from build123d import *

# Parameters (mm, degrees)
F0_R     = 3.175
F1_DEPTH = 3.048


with BuildPart() as f1:
    # F0 (on Front) → F1 (new body)
    with BuildSketch(Plane.XZ):
        with BuildLine():
            ThreePointArc((3.175, 0), (-2.2450640303, -2.2450640303), (0, 3.175))
            Line((0, 3.175), (0, 7.9375))
            ThreePointArc((0, 7.9375), (-6.000186009, 5.1963135112), (-7.8560875915, -1.1339285714))
            ThreePointArc((-7.8560875915, -1.1339285714), (-5.1963135112, -6.000186009), (0, -7.9375))
            ThreePointArc((0, -7.9375), (5.6126600757, -5.6126600757), (7.9375, 0))
            Line((7.9375, 0), (3.175, 0))
        make_face()
        with BuildLine():
            ThreePointArc((-7.8560875915, -1.1339285714), (-6.000186009, 5.1963135112), (0, 7.9375))
            Line((0, 7.9375), (0, 39.6875))
            ThreePointArc((0, 39.6875), (-10.3926270225, 43.562127982), (-15.7121751829, 53.2946428571))
            Line((-15.7121751829, 53.2946428571), (-7.8560875915, -1.1339285714))
        make_face()
        with BuildLine():
            Line((0, 39.6875), (0, 7.9375))
            ThreePointArc((0, 7.9375), (5.6126600757, 5.6126600757), (7.9375, 0))
            Line((7.9375, 0), (36.5125, 0))
            ThreePointArc((36.5125, 0), (38.8373399243, 5.6126600757), (44.45, 7.9375))
            Line((44.45, 7.9375), (18.3455357436, 7.9375))
            ThreePointArc((18.3455357436, 7.9375), (12.335749437, 10.6830723871), (10.476878412, 17.0234428571))
            Line((10.476878412, 17.0234428571), (15.7121751829, 53.2946428571))
            ThreePointArc((15.7121751829, 53.2946428571), (10.3926270225, 43.562127982), (0, 39.6875))
        make_face()
        with BuildLine():
            Line((36.5125, 0), (7.9375, 0))
            ThreePointArc((7.9375, 0), (5.6126600757, -5.6126600757), (0, -7.9375))
            Line((0, -7.9375), (44.45, -7.9375))
            ThreePointArc((44.45, -7.9375), (38.8373399243, -5.6126600757), (36.5125, 0))
        make_face()
        with BuildLine():
            ThreePointArc((-15.7121751829, 53.2946428571), (-10.3926270225, 43.562127982), (0, 39.6875))
            Line((0, 39.6875), (0, 52.3875))
            ThreePointArc((0, 52.3875), (-3.175, 55.5625), (0, 58.7375))
            Line((0, 58.7375), (0, 71.4375))
            ThreePointArc((0, 71.4375), (-10.6011956271, 67.3790255586), (-15.7819589391, 57.2787159089))
            ThreePointArc((-15.7819589391, 57.2787159089), (-15.8725653423, 55.284481195), (-15.7121751829, 53.2946428571))
        make_face()
        with BuildLine():
            Line((0, 52.3875), (0, 39.6875))
            ThreePointArc((0, 39.6875), (10.3926270225, 43.562127982), (15.7121751829, 53.2946428571))
            ThreePointArc((15.7121751829, 53.2946428571), (15.8342414727, 54.4256526112), (15.875, 55.5625))
            ThreePointArc((15.875, 55.5625), (15.8517226608, 56.4218681903), (15.7819589056, 57.2787162162))
            ThreePointArc((15.7819589056, 57.2787162162), (10.601195512, 67.3790256618), (0, 71.4375))
            Line((0, 71.4375), (0, 58.7375))
            ThreePointArc((0, 58.7375), (2.2450640303, 57.8075640303), (3.175, 55.5625))
            ThreePointArc((3.175, 55.5625), (2.2450640303, 53.3174359697), (0, 52.3875))
        make_face()
        with BuildLine():
            ThreePointArc((44.45, 7.9375), (38.8373399243, 5.6126600757), (36.5125, 0))
            ThreePointArc((36.5125, 0), (38.8373399243, -5.6126600757), (44.45, -7.9375))
            ThreePointArc((44.45, -7.9375), (50.0626600757, -5.6126600757), (52.3875, 0))
            ThreePointArc((52.3875, 0), (50.0626600757, 5.6126600757), (44.45, 7.9375))
        make_face()
        with BuildLine():
            ThreePointArc((47.625, 0), (44.45, -3.175), (41.275, 0))
            ThreePointArc((41.275, 0), (44.45, 3.175), (47.625, 0))
        make_face(mode=Mode.SUBTRACT)
        with BuildLine():
            Line((-9.4691753434, 115.3297297297), (-15.7819589391, 57.2787159089))
            ThreePointArc((-15.7819589391, 57.2787159089), (-10.6011956271, 67.3790255586), (0, 71.4375))
            Line((0, 71.4375), (0, 88.7612230935))
            Line((0, 88.7612230935), (0, 104.775))
            ThreePointArc((0, 104.775), (-7.0899153971, 107.9392826928), (-9.4691753434, 115.3297297297))
        make_face()
        with Locations((-3.175, 88.7612230935)):
            Circle(F0_R, mode=Mode.SUBTRACT)
        with BuildLine():
            Line((0, 88.7612230935), (0, 71.4375))
            ThreePointArc((0, 71.4375), (10.601195512, 67.3790256618), (15.7819589056, 57.2787162162))
            Line((15.7819589056, 57.2787162162), (9.4691753434, 115.3297297297))
            ThreePointArc((9.4691753434, 115.3297297297), (9.5110335965, 114.8156209142), (9.525, 114.3))
            ThreePointArc((9.525, 114.3), (6.7351920908, 107.5648079092), (0, 104.775))
            Line((0, 104.775), (0, 88.7612230935))
        make_face()
        with BuildLine():
            ThreePointArc((9.4691753434, 115.3297297297), (0, 123.825), (-9.4691753434, 115.3297297297))
            ThreePointArc((-9.4691753434, 115.3297297297), (-7.0899153971, 107.9392826928), (0, 104.775))
            ThreePointArc((0, 104.775), (6.7351920908, 107.5648079092), (9.525, 114.3))
            ThreePointArc((9.525, 114.3), (9.5110335965, 114.8156209142), (9.4691753434, 115.3297297297))
        make_face()
        with BuildLine():
            ThreePointArc((3.175, 114.3), (2.2450640303, 112.0549359697), (0, 111.125))
            ThreePointArc((0, 111.125), (-2.2450640303, 116.5450640303), (3.175, 114.3))
        make_face(mode=Mode.SUBTRACT)
    extrude(amount=F1_DEPTH)


solid = f1.part
The listing builds one solid part. Answer for the finished solid, in the listing's coordinates (mm). A direction names the side the tool comes from. Give positions to 0.01 mm unless a question says otherwise; leave off trailing zeros. Write each loop counter-clockwise with the first axis right and the second up, starting at its lowest first coordinate (ties: lowest second). Pieces come first, ordered by that corner, then holes. Notation, with made-up numbers: (-8.75, 72) - (-3.75, 72) arc R22 cw to (-3.75, 104) - close; hole circle Ø7 at (-25, -37). An arc over 180 degrees is marked (long way). Use a Markdown table: item, result.
1. Section D-D on x = 33.5 is taken. Write down the section's boundary in (y, z), plus the area to 3 significant figures.
Values follow:
| item | result |
|---|---|
| outline | (-3.05, -7.94) - (0, -7.94) - (0, 7.94) - (-3.05, 7.94) - close |
| area | 48.4 mm² |
2. Section A-A on x = 46 is taken. Write down the section's boundary in (y, z).
Values follow:
| item | result |
|---|---|
| outline | (-3.05, -7.78) - (0, -7.78) - (0, -2.77) - (-3.05, -2.77) - close; (-3.05, 2.77) - (0, 2.77) - (0, 7.78) - (-3.05, 7.78) - close |
3. For a pull along X with two mould halves and no side action, classify faces 1 (the flat face through (-12.58, -1.5, 86.71)), 2 (the flat face through (13.06, -1.5, 34.91)), 3 (the cylindrical face through (-2.17, -1.5, -2.32)) as released by +X, released by -X, zero draft, split by the parting line, or undercut.
Values follow:
| item | result |
|---|---|
| face 1 | released by -X |
| face 2 | released by +X |
| face 3 | undercut |
4. Section C-C on x = -1.5 is taken. Write down the section's boundary in (y, z).
Values follow:
| item | result |
|---|---|
| outline | (-3.05, -7.79) - (0, -7.79) - (0, -2.8) - (-3.05, -2.8) - close; (-3.05, 2.8) - (0, 2.8) - (0, 52.76) - (-3.05, 52.76) - close; (-3.05, 58.36) - (0, 58.36) - (0, 86.06) - (-3.05, 86.06) - close; (-3.05, 91.46) - (0, 91.46) - (0, 111.5) - (-3.05, 111.5) - close; (-3.05, 117.1) - (0, 117.1) - (0, 123.71) - (-3.05, 123.71) - close |
5. Section B-B on y = -2.1 is taken. Count the separate pieces of the cut face and the enclosed holes in it, plus the area to 3 significant figures.
Values follow:
| item | result |
|---|---|
| separate pieces | 1 |
| enclosed holes | 5 |
| area | 3,580 mm² |
6. Find the intervals of material crossed by probe 1 along Z at (x, y) = (30.5, -0.1); probe 2 along X at (y, z) = (-0.75, 114.3) (3 decimals); probe 3 along Z at (x, y) = (6, -2.4), in increasing order. Write a range as from..to.
Values follow:
| item | result |
|---|---|
| probe 1 | z = -7.94..7.94 |
| probe 2 | x = -9.581..-3.175, 3.175..9.581 |
| probe 3 | z = -7.94..0, 5.2..121.7 |
7. Each of these flat-tipped pins is pushed along its axis until it touches: P1, Ø0.9, axis at x = 35.5, y = -1, coming from the +Z side; P2, Ø1.5, axis at x = 6.5, y = -1.5, coming from the +Z side. Where does it stop, or does it pass through?
Values follow:
| item | result |
|---|---|
| P1 | stops at z = 7.94 |
| P2 | stops at z = 121.89 |
8. A tool of negligible diameter and unlimited length cuts with its end or side. For faces 4 (the flat face through (6, -2, 0)), 5 (the flat face through (32, -2, 7.938)), 6 (the cylindrical face through (12.4, -1.5, 10.61)), from which of +Z, -Z, +X, -X, +Y, -Y can it reach the whole face along a straight path? Write none if from no direction.
Values follow:
| item | result |
|---|---|
| face 4 | +Y, -Y |
| face 5 | +Z, +X, +Y, -Y |
| face 6 | +X, +Y, -Y |
